For this review, take the finished solid that the model builds, in its own axes (mm). Face numbers are marked on the shaded views. A direction names the side the tool comes from. Give positions to 0.01 mm unless a question says otherwise; leave off trailing zeros. Write each loop counter-clockwise with the first axis right and the second up, starting at its lowest first coordinate (ties: lowest second). Pieces come first, ordered by that corner, then holes.
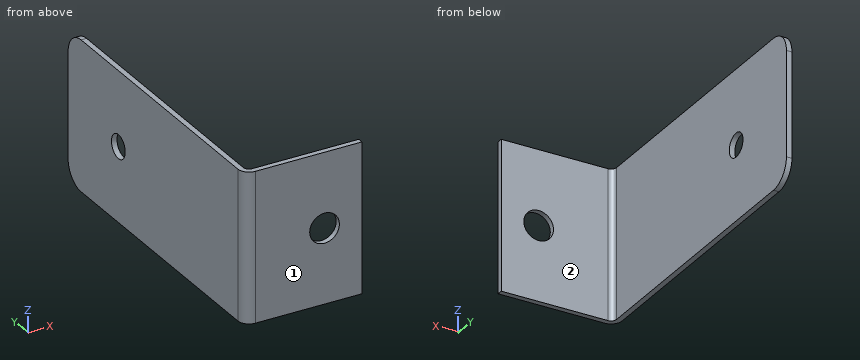
from build123d import *

# Parameters (mm, degrees)
BASE_FLANGE1_DEPTH      = 10
BASE_FLANGE1_DEPTH_BACK = 10
SKETCH6_R               = 1.5875
CUT_EXTRUDE1_DEPTH      = 10
SKETCH7_R               = 1.984375
CUT_EXTRUDE2_DEPTH      = 10
FILLET1_R               = 3


# Sheet-metal steps are written as plain solids
with BuildPart() as part:
    # Sketch1 → Base-Flange1 (new, two sides: drawn at the far end of the back side and taken through both)
    with BuildSketch(Plane.XY.offset(-BASE_FLANGE1_DEPTH_BACK)):
        with BuildLine():
            Line((0, 40), (0, 0.7366))
            ThreePointArc((0, 0.7366), (0.215745145, 0.215745145), (0.7366, 0))
            Line((0.7366, 0), (15, 0))
            Line((15, 0), (15, -0.7366))
            Line((15, -0.7366), (0.7366, -0.7366))
            ThreePointArc((0.7366, -0.7366), (-0.30510971, -0.30510971), (-0.7366, 0.7366))
            Line((-0.7366, 0.7366), (-0.7366, 40))
            Line((-0.7366, 40), (0, 40))
        make_face()
    extrude(amount=BASE_FLANGE1_DEPTH + BASE_FLANGE1_DEPTH_BACK)

    # Sketch6 → Cut-Extrude1 (cut)
    with BuildSketch(Plane(origin=(0, 0, 0), x_dir=(0, 0, -1), z_dir=(1, 0, 0))):
        with Locations(Location((0, 28.3734, 0), (0, 0, 90))):
            Circle(SKETCH6_R)
    extrude(amount=-CUT_EXTRUDE1_DEPTH, mode=Mode.SUBTRACT)

    # Sketch7 → Cut-Extrude2 (cut)
    with BuildSketch(Plane(origin=(0, 0, 0), x_dir=(1, 0, 0), z_dir=(0, 1, 0))):
        with Locations(Location((10, 0, 0), (0, 0, 270))):
            Circle(SKETCH7_R)
    extrude(amount=-CUT_EXTRUDE2_DEPTH, mode=Mode.SUBTRACT)

    # Fillet1
    fillet1_edges = [part.edges().sort_by_distance(p)[0] for p in [
        (-0.3683, 40, 10),
        (-0.3683, 40, -10),
    ]]
    fillet(fillet1_edges, radius=FILLET1_R)


solid = part.part
(1) Tool access review of the marked faces 1 and 2: name each direction out of +Z, -Z, +X, -X, +Y, -Y from which nothing blocks a thin tool from reaching the whole face with its end or side.
(2) Clearance check with flat-ended pins moving along their axes: pin 1 Ø6 at (y, z) = (21.5, -3) entering from +X; pin 2 Ø4.5 at (x, z) = (8, -4.5) entering from +Y. State where each tip first meets the part, or that it passes through.
(3) We need section A-A (z = 0). Write out the cut boundary in (x, y), and give its area (3 significant figures).
(4) We need section B-B (x = 10). Write out the cut boundary in (y, z), and give its area (3 significant figures).
(5) We need section C-C (z = -6.25). Write out the cut boundary in (x, y).
(6) We need section D-D (y = 3.5). Write out the cut boundary in (x, z).
(7) For L1, parallel to Y at x = 8.5, z = -8; L2, parallel to X at y = -0.45, z = 0, list the stretches that pass through material, from the lowest coordinate up.
The answers:
1. face 1: +Z, -Z, +X, -X, -Y
1. face 2: +Z, -Z, +X, +Y
2. pin 1: stops at x = 0
2. pin 2: stops at y = 0
3. outline: (-0.74, 0.74) arc R1.47 ccw to (0.74, -0.74) - (8.02, -0.74) - (8.02, 0) - (0.74, 0) arc R0.74 cw to (0, 0.74) - (0, 26.79) - (-0.74, 26.79) - close; (-0.74, 29.96) - (0, 29.96) - (0, 40) - (-0.74, 40) - close; (11.98, -0.74) - (15, -0.74) - (15, 0) - (11.98, 0) - close
3. area: 35.4 mm2
4. outline: (-0.74, -10) - (0, -10) - (0, -1.98) - (-0.74, -1.98) - close; (-0.74, 1.98) - (0, 1.98) - (0, 10) - (-0.74, 10) - close
4. area: 11.8 mm2
5. outline: (-0.74, 0.74) arc R1.47 ccw to (0.74, -0.74) - (15, -0.74) - (15, 0) - (0.74, 0) arc R0.74 cw to (0, 0.74) - (0, 40) - (-0.74, 40) - close
6. outline: (-0.74, -10) - (0, -10) - (0, 10) - (-0.74, 10) - close
7. L1: y = -0.74 to 0
7. L2: x = -0.14 to 8.02, 11.98 to 15
